Here's how the part is built. I have some questions about the finished solid (model axes, mm). Round coordinates to 2 decimals unless told otherwise and drop trailing zeros. Write each loop counter-clockwise with the first axis right and the second up, starting at its lowest first coordinate (ties: lowest second). Pieces come first, ordered by that corner, then holes. Notation, with made-up numbers: (-35.5, 18) -> (-13.5, 18) arc R22 cw to (-13.5, 35) -> close; hole circle Ø11 at (51.25, 32.25). An arc over 180 degrees is marked (long way). Put each result on its own line as item: value. Start each with the question number.
1) I want a section at C-C, the plane y = 20. List the corners of the cut face in (x, z) for me, then the cut area to 3 significant figures.
2) If I drill on line 1 along Y through (x, z) = (-14.35, 0.75); line 2 along Y through (x, z) = (0, 1.5); line 3 along Y through (x, z) = (9.5, 0.45), over which ranges is the centre line in solid material (lowest first)? Write a range as [from, to].
3) I want a section at D-D, the plane x = -33.5. List the corners of the cut face in (y, z) for me, then the cut area to 3 significant figures.
4) I want a section at B-B, the plane y = 7. List the corners of the cut face in (x, z) for me, then the cut area to 3 significant figures.
5) Will these pins go through, and if not, where does the flat tip stop? P1, Ø1, axis at x = 33, z = 0.5, coming from the +Y side; P2, Ø0.6, axis at y = -26, z = 1, coming from the -X side; P3, Ø0.6, axis at y = 27, z = 0.5, coming from the +X side.
6) I want a section at A-A, the plane x = -14.35. List the corners of the cut face in (y, z) for me, then the cut area to 3 significant figures.
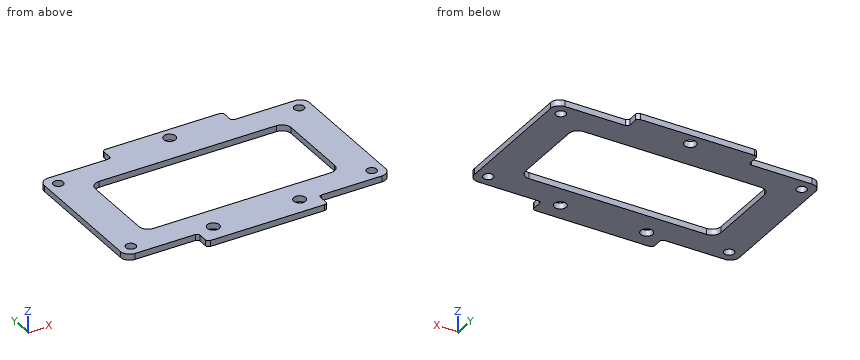
from build123d import *

# Parameters (mm, degrees)
SKETCH_1_W          = 88
SKETCH_1_H          = 48
SKETCH_1_R          = 1.65
EXTRUDE_1_DEPTH     = 2
FILLET_1_R          = 3
SKETCH_3_W          = 40
SKETCH_3_H          = 10
EXTRUDE_2_DEPTH     = 2
SKETCH_2_R          = 2
CUT_EXTRUDE_1_DEPTH = 2
SKETCH_4_W          = 65
SKETCH_4_H          = 30
CUT_EXTRUDE_2_DEPTH = 2
FILLET_2_R          = 3
FILLET_3_R          = 1


with BuildPart() as part:
    # 草图1 → 凸台-拉伸1 (new body)
    with BuildSketch(Plane.XY):
        Rectangle(SKETCH_1_W, SKETCH_1_H)
        with Locations((-40, 20)):
            Circle(SKETCH_1_R, mode=Mode.SUBTRACT)
        with Locations((40, 20)):
            Circle(SKETCH_1_R, mode=Mode.SUBTRACT)
        with Locations((40, -20)):
            Circle(SKETCH_1_R, mode=Mode.SUBTRACT)
        with Locations((-40, -20)):
            Circle(SKETCH_1_R, mode=Mode.SUBTRACT)
    extrude(amount=EXTRUDE_1_DEPTH)

    # 圆角1
    fillet_1_edges = [part.edges().sort_by_distance(p)[0] for p in [
        (-44, 24, 1),
        (44, 24, 1),
        (44, -24, 1),
        (-44, -24, 1),
    ]]
    fillet(fillet_1_edges, radius=FILLET_1_R)

    # 草图3 → 凸台-拉伸2 (add)
    with BuildSketch(Plane.XY.offset(2)):
        with Locations((0, 24)):
            Rectangle(SKETCH_3_W, SKETCH_3_H)
        with Locations((0, -24)):
            Rectangle(SKETCH_3_W, SKETCH_3_H)
    extrude(amount=-EXTRUDE_2_DEPTH)

    # 草图2 → 切除-拉伸1 (cut)
    with BuildSketch(Plane.XY.offset(2)):
        with Locations((0, 25)):
            Circle(SKETCH_2_R)
        with Locations((-14.35, -22.896529102)):
            Circle(SKETCH_2_R)
        with Locations((14.35, -22.896529102)):
            Circle(SKETCH_2_R)
    extrude(amount=-CUT_EXTRUDE_1_DEPTH, mode=Mode.SUBTRACT)

    # 草图4 → 切除-拉伸2 (cut)
    with BuildSketch(Plane.XY.offset(2)):
        Rectangle(SKETCH_4_W, SKETCH_4_H)
    extrude(amount=-CUT_EXTRUDE_2_DEPTH, mode=Mode.SUBTRACT)

    # 圆角2
    fillet_2_edges = [part.edges().sort_by_distance(p)[0] for p in [
        (-32.5, -15, 1),
        (-32.5, 15, 1),
        (32.5, 15, 1),
        (32.5, -15, 1),
    ]]
    fillet(fillet_2_edges, radius=FILLET_2_R)

    # 圆角3
    fillet_3_edges = [part.edges().sort_by_distance(p)[0] for p in [
        (20, 24, 1),
        (-20, 24, 1),
        (20, 29, 1),
        (-20, 29, 1),
        (20, -24, 1),
        (-20, -24, 1),
        (-20, -29, 1),
        (20, -29, 1),
    ]]
    fillet(fillet_3_edges, radius=FILLET_3_R)


solid = part.part
Findings:
1. outline: (-44, 0) -> (-41.65, 0) -> (-41.65, 2) -> (-44, 2) -> close; (-38.35, 0) -> (38.35, 0) -> (38.35, 2) -> (-38.35, 2) -> close; (41.65, 0) -> (44, 0) -> (44, 2) -> (41.65, 2) -> close
1. area: 163 mm2
2. line 1: y = [-29, -24.9], [-20.9, -15], [15, 29]
2. line 2: y = [-29, -15], [15, 23], [27, 29]
2. line 3: y = [-29, -15], [15, 29]
3. outline: (-24, 0) -> (24, 0) -> (24, 2) -> (-24, 2) -> close
3. area: 96.0 mm2
4. outline: (-44, 0) -> (-32.5, 0) -> (-32.5, 2) -> (-44, 2) -> close; (32.5, 0) -> (44, 0) -> (44, 2) -> (32.5, 2) -> close
4. area: 46.0 mm2
5. P1: stops at y = 24
5. P2: stops at x = -20
5. P3: stops at x = 20
6. outline: (-29, 0) -> (-24.9, 0) -> (-24.9, 2) -> (-29, 2) -> close; (-20.9, 0) -> (-15, 0) -> (-15, 2) -> (-20.9, 2) -> close; (15, 0) -> (29, 0) -> (29, 2) -> (15, 2) -> close
6. area: 48.0 mm2
